Here's the drawing with two shaded views (mm, measured from the low corner). I have some questions. A direction names the side the tool comes from. Coordinates: 2 decimals unless noted, no trailing zeros. Loops run counter-clockwise (first coordinate to the right, second up) from the corner with the lowest first, then second, coordinate; pieces in that order, holes last. Notation, with made-up numbers: (-19.5, 87) - (9.5, 87) arc R18 cw to (9.5, 103) - close; hole circle Ø5 at (69, -35.75). An arc over 180 degrees is marked (long way). Use a Markdown table: item, result.
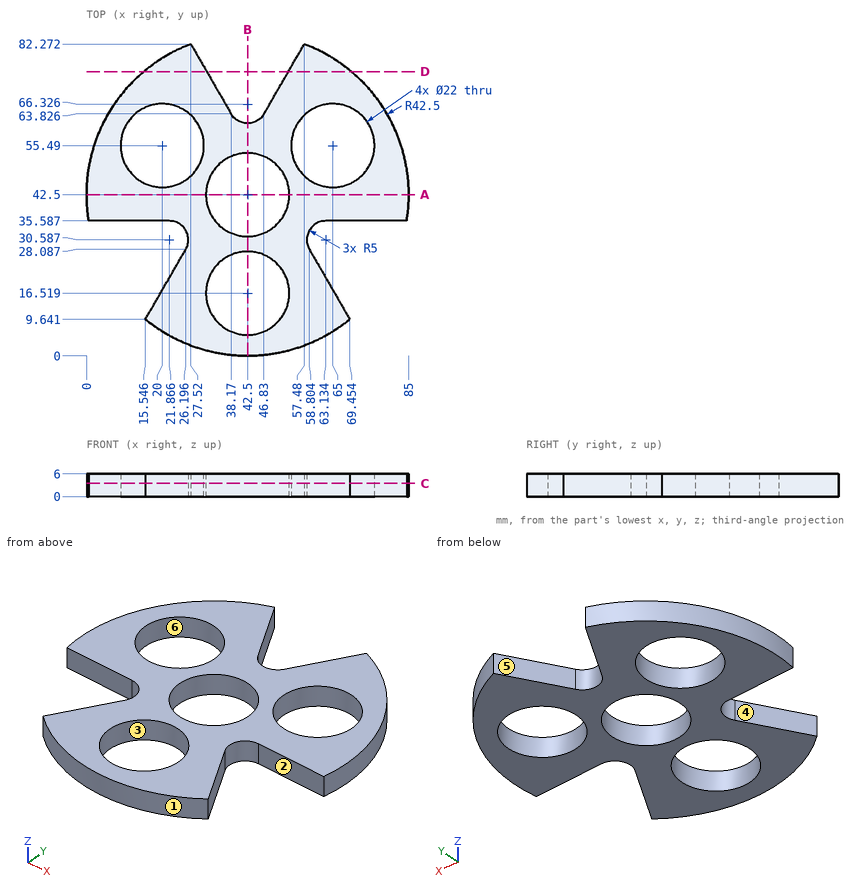
Q1. If we mould it in two halves opening along X, with no side actions, what happens to the marked faces 1, 2 and 3? For each: pulls with the +X half, pulls with the -X half, needs draft (parallel to the pull), parting line crosses it, or undercut.
Check values:
| item | result |
|---|---|
| face 1 | parting line crosses it |
| face 2 | needs draft |
| face 3 | undercut |
Q2. Which directions (+Z, -Z, +X, -X, +Y, -Y) give clear straight access to the entire face, cutting with the end or side of a thin tool? Please do the marked faces 4, 5 and 6.
Check values:
| item | result |
|---|---|
| face 4 | +Z, -Z, -X |
| face 5 | +Z, -Z, +Y |
| face 6 | +Z, -Z |
Q3. I want a section at D-D, the plane y = 75. Write out the boundary of the cut face in (x, z), then the cut area to 3 significant figures.
Check values:
| item | result |
|---|---|
| outline | (15.11, 0) - (31.72, 0) - (31.72, 6) - (15.11, 6) - close; (53.28, 0) - (69.89, 0) - (69.89, 6) - (53.28, 6) - close |
| area | 199 mm^2 |
Q4. Please list where these lines run through material, in increasing order: L1, parallel to Y at x = 44, z = 2 (1 decimal); L2, parallel to Y at x = 36, z = 2.5 (1 decimal); L3, parallel to X at y = 56, z = 1. Write a range as from..to.
Check values:
| item | result |
|---|---|
| L1 | 0..5.6, 27.4..31.6, 53.4..61.6 |
| L2 | 0.5..7.6, 25.4..33.6, 51.4..67.6 |
| L3 | 2.2..9.01, 30.99..54.01, 75.99..82.8 |
Q5. Will these pins go through, and if not, where does the flat tip stop? P1, Ø1.8, axis at x = 68.5, z = 4, coming from the -Y side (1 decimal); P2, Ø13, axis at x = 65, y = 55.49, coming from the +Z side; P3, Ø2, axis at x = 49, z = 4, coming from the +Y side (1 decimal); P4, Ø3, axis at y = 64.5, z = 3, coming from the +X side.
Check values:
| item | result |
|---|---|
| P1 | y = 8.2 |
| P2 | through |
| P3 | y = 69.3 |
| P4 | x = 79.73 |
Q6. I want a section at C-C, the plane z = 3.5. Write out the boundary of the cut face in (x, y) (1 decimal).
Check values:
| item | result |
|---|---|
| outline | (0.6, 35.6) - (21.9, 35.6) arc R5 cw to (26.2, 28.1) - (15.5, 9.6) arc R42.5 ccw to (69.5, 9.6) - (58.8, 28.1) arc R5 cw to (63.1, 35.6) - (84.4, 35.6) arc R42.5 ccw to (57.5, 82.3) - (46.8, 63.8) arc R5 cw to (38.2, 63.8) - (27.5, 82.3) arc R42.5 ccw to start; hole circle Ø22 at (20, 55.5); hole circle Ø22 at (42.5, 16.5); hole circle Ø22 at (42.5, 42.5); hole circle Ø22 at (65, 55.5) |
Q7. I want a section at B-B, the plane x = 42.5. Write out the boundary of the cut face in (y, z) (1 decimal), then the cut area to 3 significant figures.
Check values:
| item | result |
|---|---|
| outline | (0, 0) - (5.5, 0) - (5.5, 6) - (0, 6) - close; (27.5, 0) - (31.5, 0) - (31.5, 6) - (27.5, 6) - close; (53.5, 0) - (61.3, 0) - (61.3, 6) - (53.5, 6) - close |
| area | 104 mm^2 |
Q8. I want a section at A-A, the plane y = 42.5. Write out the boundary of the cut face in (x, z), then the cut area to 3 significant figures.
Check values:
| item | result |
|---|---|
| outline | (0, 0) - (31.5, 0) - (31.5, 6) - (0, 6) - close; (53.5, 0) - (85, 0) - (85, 6) - (53.5, 6) - close |
| area | 378 mm^2 |
